```python
from build123d import *

# Parameters (mm, degrees)
SKETCH1_W           = 214.108538
SKETCH1_H           = 214.108538
SKETCH1_R           = 2.0701
BOSS_EXTRUDE1_DEPTH = 1.5875
SKETCH2_W           = 38.371842409
SKETCH2_H           = 38.371842409
SKETCH2_H_2         = 35.196842409
SKETCH2_W_2         = 35.196842409
CUT_EXTRUDE1_DEPTH  = 152.405921874
FILLET1_R           = 3.175
FILLET2_R           = 3.175


with BuildPart() as part:
    # Sketch1 → Boss-Extrude1 (new body)
    with BuildSketch(Plane(origin=(0, 0, 0), x_dir=(1, 0, 0), z_dir=(0, 1, 0))):
        Rectangle(SKETCH1_W, SKETCH1_H)
        with Locations(Location((-101.809169, 101.809169, 0), (0, 0, 270))):
            Circle(SKETCH1_R, mode=Mode.SUBTRACT)
        with Locations(Location((-101.809169, -101.809169, 0), (0, 0, 270))):
            Circle(SKETCH1_R, mode=Mode.SUBTRACT)
        with Locations(Location((101.809169, -101.809169, 0), (0, 0, 270))):
            Circle(SKETCH1_R, mode=Mode.SUBTRACT)
        with Locations(Location((101.809169, 101.809169, 0), (0, 0, 270))):
            Circle(SKETCH1_R, mode=Mode.SUBTRACT)
        with Locations(Location((-88.338784818, 88.338784818, 0), (0, 0, 270))):
            Circle(SKETCH1_R, mode=Mode.SUBTRACT)
        with Locations(Location((88.338784818, -88.338784818, 0), (0, 0, 90))):
            Circle(SKETCH1_R, mode=Mode.SUBTRACT)
        with Locations(Location((88.338784818, 88.338784818, 0), (0, 0, 270))):
            Circle(SKETCH1_R, mode=Mode.SUBTRACT)
        with Locations(Location((-88.338784818, -88.338784818, 0), (0, 0, 90))):
            Circle(SKETCH1_R, mode=Mode.SUBTRACT)
    extrude(amount=BOSS_EXTRUDE1_DEPTH)

    # Sketch2 → Cut-Extrude1 (cut, through all)
    with BuildSketch(Plane(origin=(0, 1.5875, 0), x_dir=(1, 0, 0), z_dir=(0, 1, 0))):
        with Locations((-63.907763614, 63.907763614)):
            Rectangle(SKETCH2_W, SKETCH2_H)
        with Locations((-63.907763614, 20.773421204)):
            Rectangle(SKETCH2_W, SKETCH2_H_2)
        with Locations((-20.773421204, 63.907763614)):
            Rectangle(SKETCH2_W_2, SKETCH2_H)
        with Locations((-20.773421204, 20.773421204)):
            Rectangle(SKETCH2_W_2, SKETCH2_H_2)
        with Locations((20.773421204, 63.907763614)):
            Rectangle(SKETCH2_W_2, SKETCH2_H)
        with Locations((20.773421204, 20.773421204)):
            Rectangle(SKETCH2_W_2, SKETCH2_H_2)
        with Locations((63.907763614, 63.907763614)):
            Rectangle(SKETCH2_W, SKETCH2_H)
        with Locations((63.907763614, 20.773421204)):
            Rectangle(SKETCH2_W, SKETCH2_H_2)
        with Locations((63.907763614, -20.773421204)):
            Rectangle(SKETCH2_W, SKETCH2_H_2)
        with Locations((20.773421204, -20.773421204)):
            Rectangle(SKETCH2_W_2, SKETCH2_H_2)
        with Locations((-20.773421204, -20.773421204)):
            Rectangle(SKETCH2_W_2, SKETCH2_H_2)
        with Locations((-63.907763614, -20.773421204)):
            Rectangle(SKETCH2_W, SKETCH2_H_2)
        with Locations((-63.907763614, -63.907763614)):
            Rectangle(SKETCH2_W, SKETCH2_H)
        with Locations((-20.773421204, -63.907763614)):
            Rectangle(SKETCH2_W_2, SKETCH2_H)
        with Locations((20.773421204, -63.907763614)):
            Rectangle(SKETCH2_W_2, SKETCH2_H)
        with Locations((63.907763614, -63.907763614)):
            Rectangle(SKETCH2_W, SKETCH2_H)
    extrude(amount=-CUT_EXTRUDE1_DEPTH, mode=Mode.SUBTRACT)

    # Fillet1
    fillet1_edges = [part.edges().sort_by_distance(p)[0] for p in [
        (-107.054269, 0.79375, -107.054269),
        (107.054269, 0.79375, -107.054269),
        (107.054269, 0.79375, 107.054269),
        (-107.054269, 0.79375, 107.054269),
    ]]
    fillet(fillet1_edges, radius=FILLET1_R)

    # Fillet2
    fillet2_edges = [part.edges().sort_by_distance(p)[0] for p in [
        (-44.721842409, 0.79375, -44.721842409),
        (-83.093684818, 0.79375, -44.721842409),
        (-83.093684818, 0.79375, -83.093684818),
        (-44.721842409, 0.79375, -83.093684818),
        (-44.721842409, 0.79375, -38.371842409),
        (-44.721842409, 0.79375, -3.175),
        (-83.093684818, 0.79375, -3.175),
        (-83.093684818, 0.79375, -38.371842409),
        (-3.175, 0.79375, -83.093684818),
        (-3.175, 0.79375, -44.721842409),
        (-38.371842409, 0.79375, -44.721842409),
        (-38.371842409, 0.79375, -83.093684818),
        (-3.175, 0.79375, -38.371842409),
        (-3.175, 0.79375, -3.175),
        (-38.371842409, 0.79375, -3.175),
        (-38.371842409, 0.79375, -38.371842409),
        (38.371842409, 0.79375, -44.721842409),
        (3.175, 0.79375, -44.721842409),
        (3.175, 0.79375, -83.093684818),
        (38.371842409, 0.79375, -83.093684818),
        (38.371842409, 0.79375, -3.175),
        (3.175, 0.79375, -3.175),
        (3.175, 0.79375, -38.371842409),
        (38.371842409, 0.79375, -38.371842409),
        (44.721842409, 0.79375, -44.721842409),
        (44.721842409, 0.79375, -83.093684818),
        (83.093684818, 0.79375, -83.093684818),
        (83.093684818, 0.79375, -44.721842409),
        (83.093684818, 0.79375, -38.371842409),
        (83.093684818, 0.79375, -3.175),
        (44.721842409, 0.79375, -3.175),
        (44.721842409, 0.79375, -38.371842409),
        (44.721842409, 0.79375, 38.371842409),
        (44.721842409, 0.79375, 3.175),
        (83.093684818, 0.79375, 3.175),
        (83.093684818, 0.79375, 38.371842409),
        (38.371842409, 0.79375, 38.371842409),
        (3.175, 0.79375, 38.371842409),
        (3.175, 0.79375, 3.175),
        (38.371842409, 0.79375, 3.175),
        (-3.175, 0.79375, 3.175),
        (-3.175, 0.79375, 38.371842409),
        (-38.371842409, 0.79375, 38.371842409),
        (-38.371842409, 0.79375, 3.175),
        (-44.721842409, 0.79375, 38.371842409),
        (-83.093684818, 0.79375, 38.371842409),
        (-83.093684818, 0.79375, 3.175),
        (-44.721842409, 0.79375, 3.175),
        (-44.721842409, 0.79375, 44.721842409),
        (-44.721842409, 0.79375, 83.093684818),
        (-83.093684818, 0.79375, 83.093684818),
        (-83.093684818, 0.79375, 44.721842409),
        (-3.175, 0.79375, 44.721842409),
        (-3.175, 0.79375, 83.093684818),
        (-38.371842409, 0.79375, 83.093684818),
        (-38.371842409, 0.79375, 44.721842409),
        (38.371842409, 0.79375, 83.093684818),
        (3.175, 0.79375, 83.093684818),
        (3.175, 0.79375, 44.721842409),
        (38.371842409, 0.79375, 44.721842409),
        (83.093684818, 0.79375, 44.721842409),
        (83.093684818, 0.79375, 83.093684818),
        (44.721842409, 0.79375, 83.093684818),
        (44.721842409, 0.79375, 44.721842409),
    ]]
    fillet(fillet2_edges, radius=FILLET2_R)


solid = part.part
```
Here's how the part is built. I have some questions about the finished solid (model axes, mm). Coordinates: 2 decimals unless noted, no trailing zeros. Order: outer loops, then holes, each group sorted by start corner. A loop starts at its lowest first (then second) coordinate and runs counter-clockwise, first axis right, second up. Notation, with made-up numbers: (12.25, 45.5) -> (59.25, 45.5) arc R8 cw to (59.25, 54.5) -> close; hole circle Ø2 at (42.5, 13.25). An arc over 180 degrees is marked (long way). Return JSON: item names as keys, results as strings.
1) If we section it at A-A on z = 17: List the corners of the cut face in (x, y) for me (1 decimal), plus the area to 3 significant figures.
Conclusion:
{"outline": "(-107.1, 0) -> (-83.1, 0) -> (-83.1, 1.6) -> (-107.1, 1.6) -> close; (-44.7, 0) -> (-38.4, 0) -> (-38.4, 1.6) -> (-44.7, 1.6) -> close; (-3.2, 0) -> (3.2, 0) -> (3.2, 1.6) -> (-3.2, 1.6) -> close; (38.4, 0) -> (44.7, 0) -> (44.7, 1.6) -> (38.4, 1.6) -> close; (83.1, 0) -> (107.1, 0) -> (107.1, 1.6) -> (83.1, 1.6) -> close", "area": "106 mm²"}
2) I'm going to push a flat-ended pin straight in: P1, Ø3.5, axis at x = 88.34, z = 88.34, coming from the +Y side. Where does the tip first touch, or does it pass through?
Conclusion:
{"P1": "passes through"}
3) If we section it at B-B on x = 73.5: List the corners of the cut face in (y, z) for me (1 decimal).
Conclusion:
{"outline": "(0, -107.1) -> (1.6, -107.1) -> (1.6, -83.1) -> (0, -83.1) -> close; (0, -44.7) -> (1.6, -44.7) -> (1.6, -38.4) -> (0, -38.4) -> close; (0, -3.2) -> (1.6, -3.2) -> (1.6, 3.2) -> (0, 3.2) -> close; (0, 38.4) -> (1.6, 38.4) -> (1.6, 44.7) -> (0, 44.7) -> close; (0, 83.1) -> (1.6, 83.1) -> (1.6, 107.1) -> (0, 107.1) -> close"}
4) If I drill on probe 1 along Z at (x, y) = (32, 1.05) (3 decimals); probe 2 along Z at (x, y) = (-81, 1.05), over which ranges is the centre line in solid material (lowest first)?
Conclusion:
{"probe 1": "z = -107.054 to -83.094, -44.722 to -38.372, -3.175 to 3.175, 38.372 to 44.722, 83.094 to 107.054", "probe 2": "z = -107.05 to -82.9, -44.91 to -38.18, -3.36 to 3.36, 38.18 to 44.91, 82.9 to 107.05"}
5) If we section it at C-C on y = 0.95: State how many separate pieces and enclosed holes the cut face has, plus the area to 3 significant figures.
Conclusion:
{"separate pieces": "1", "enclosed holes": "24", "area": "24,200 mm²"}
